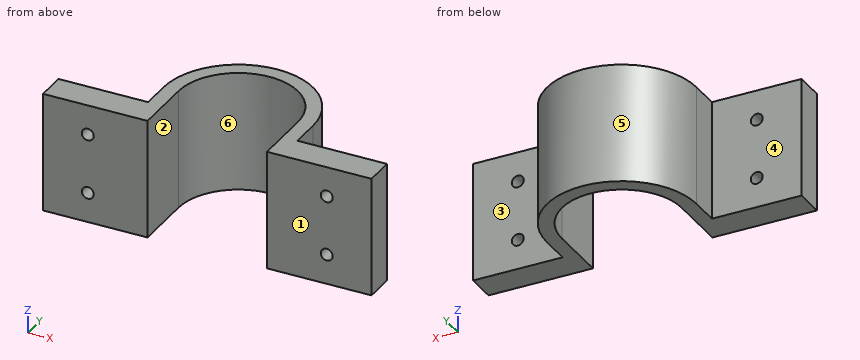
Autodesk Inventor part; units mm, degrees
ref_plane "YZ Plane" through (0, 0, 0) normal (1, 0, 0) x (0, 1, 0)
ref_plane "XZ Plane" through (0, 0, 0) normal (0, 1, 0) x (-1, 0, 0)
ref_plane "XY Plane" through (0, 0, 0) normal (0, 0, 1) x (1, 0, 0)
sketch "Sketch1" plane through (0, 0, 0) normal (0, 0, 1) x (1, 0, 0)
  arc A0 (20, 20) -> (-20, 20) centre (0, 20) ccw
  line L0 (55, 0) -> (55, 10)
  line L1 (-55, 10) -> (-55, 0)
  line L2 (55, 10) -> (25, 10)
  line L3 (-25, 10) -> (-55, 10)
  line L4 (20, 20) -> (20, 0)
  line L5 (-20, 20) -> (-20, 0)
  line L6 (25, 20) -> (25, 10)
  line L7 (-25, 20) -> (-25, 10)
  arc A1 (25, 20) -> (-25, 20) centre (0, 20) ccw
  line L8 (-55, 0) -> (-20, 0)
  line L9 (20, 0) -> (55, 0)
  point P0 (0, 0)
  dimension "d1" = 10
  dimension "d4" = 55
  dimension "d5" = 30
  dimension "d6" = 30
  dimension "d7" = 55
extrude "Extrusion1" add sketch "Sketch1" along normal blind 40
sketch "Sketch2" plane through (25, 10, 0) normal (0, 1, 0) x (1, 0, 0)
  point P0 (-25, 0)
sketch "Sketch3" plane through (25, 10, 0) normal (0, 1, 0) x (1, 0, 0)
  line L0 (30, 0) -> (0, 0) construction
  line L1 (15, 0) -> (15, -40) construction
  line L2 (30, -40) -> (0, -40) construction
  line L3 (30, 0) -> (30, -40) construction
  line L4 (30, -20) -> (-80, -20) construction
  line L5 (-80, 0) -> (-80, -40) construction
  line L6 (-50, 0) -> (-80, 0) construction
  line L7 (-65, 0) -> (-65, -40) construction
  line L8 (-50, -40) -> (-80, -40) construction
  line L9 (-80, -10) -> (30, -10) construction
  line L10 (-80, -30) -> (30, -30) construction
  circle A0 centre (15, -10) radius 2
  circle A1 centre (15, -30) radius 2
  circle A2 centre (-65, -10) radius 2
  circle A3 centre (-65, -30) radius 2
  point P0 (-25, 0)
  dimension "d8" = 4
  dimension "d9" = 4
  dimension "d10" = 4
  dimension "d11" = 4
extrude "Extrusion2" cut sketch "Sketch3" against normal blind 10
thread "Thread1"
thread "Thread2"
thread "Thread3"
thread "Thread4"
properties part number "U-bracket"
Model file for the job. Use its own axes, mm. Face numbers are marked on the shaded views. A direction names the side the tool comes from. Round coordinates to 2 decimals unless told otherwise and drop trailing zeros. Loops run counter-clockwise (first coordinate to the right, second up) from the corner with the lowest first, then second, coordinate; pieces in that order, holes last. Notation, with made-up numbers: M -29,25 L 10,25 A29 cw 10,64 Z; hole C -15.75,45 d5. An arc over 180 degrees is marked long. Put each result on its own line as item: value. Start each with the question number.
Item 1: Drop flat-ended pins along their axis: P1, Ø10, axis at x = -42, z = 19, coming from the +Y side; P2, Ø12, axis at x = -7.5, z = 9.5, coming from the +Y side; P3, Ø5, axis at y = 16.5, z = 14.5, coming from the -X side. Give the stop position or say it passes through.
Item 2: 3-axis set-ups, long thin cutter, end or side, ignore diameter. For the marked faces 1, 2 and 3: which of +Z, -Z, +X, -X, +Y, -Y reach the whole face in a straight line?
Item 3: Cut at B-B (x = 40). List the corners of the cut face in (y, z).
Item 4: Cut at D-D (z = 26.5). List the corners of the cut face in (x, y), then the cut area to 3 significant figures.
Item 5: Cut at A-A (y = 12.5). List the corners of the cut face in (x, z).
Item 6: Mould opens along X. For the marked faces 4, 5 and 6 say: released by +X, released by -X, zero draft, split by the parting line, or undercut.
Item 7: Drill centre lines: line 1 along Z through (x, y) = (40, 5.25); line 2 along X through (y, z) = (3.5, 10); line 3 along X through (y, z) = (19, 16). Where is each one in solid material? Low to high.
Item 8: Cut at C-C (z = 10). List the corners of the cut face in (x, y).
Answer block:
1. P1: y = 10
1. P2: y = 44.95
1. P3: x = -25
2. face 1: +Z, -Z, +X, -X, -Y
2. face 2: +Z, -Z, -Y
2. face 3: +Z, -Z, +X, +Y
3. outline: M 0,0 L 10,0 L 10,8 L 0,8 Z; M 0,12 L 10,12 L 10,28 L 0,28 Z; M 0,32 L 10,32 L 10,40 L 0,40 Z
4. outline: M -55,0 L -20,0 L -20,20 A20 cw 20,20 L 20,0 L 55,0 L 55,10 L 25,10 L 25,20 A25 ccw -25,20 L -25,10 L -55,10 Z
4. area: 1,150 mm2
5. outline: M -25,0 L -20,0 L -20,40 L -25,40 Z; M 20,0 L 25,0 L 25,40 L 20,40 Z
6. face 4: zero draft
6. face 5: split by the parting line
6. face 6: undercut
7. line 1: 0 to 8, 12 to 28, 32 to 40
7. line 2: -55 to -42, -38 to -20, 20 to 38, 42 to 55
7. line 3: -25 to -20, 20 to 25
8. outline: M -55,0 L -42,0 L -42,10 L -55,10 Z; M -38,0 L -20,0 L -20,20 A20 cw 20,20 L 20,0 L 38,0 L 38,10 L 25,10 L 25,20 A25 ccw -25,20 L -25,10 L -38,10 Z; M 42,0 L 55,0 L 55,10 L 42,10 Z
